```python
from build123d import *

# Parameters (mm, degrees)
BOSS_EXTRUDE1_DEPTH = 15
SKETCH3_R           = 1.5
CUT_EXTRUDE1_DEPTH  = 15


with BuildPart() as part:
    # Sketch2 → Boss-Extrude1 (new body)
    with BuildSketch(Plane(origin=(0, 0, 0), x_dir=(0, 0, -1), z_dir=(1, 0, 0))):
        with BuildLine():
            Line((8, 11.4), (-7.814981045, 11.4))
            Line((-7.814981045, 11.4), (-11.814981045, 11.4))
            Line((-11.814981045, 11.4), (-11.814981045, 9.4))
            Line((-11.814981045, 9.4), (-8, 9.4))
            Line((-8, 9.4), (-8, 0))
            ThreePointArc((-8, 0), (0, -8), (8, 0))
            Line((8, 0), (8, 9.4))
            Line((8, 9.4), (12, 9.4))
            Line((12, 9.4), (12, 11.4))
            Line((12, 11.4), (8, 11.4))
        make_face()
        with BuildLine():
            ThreePointArc((4, 0), (0, -4), (-4, 0))
            ThreePointArc((-4, 0), (0, 4), (4, 0))
        make_face(mode=Mode.SUBTRACT)
    extrude(amount=BOSS_EXTRUDE1_DEPTH)

    # Sketch3 → Cut-Extrude1 (cut)
    with BuildSketch(Plane.XZ.offset(-9.4)):
        with Locations(Location((2.464362638, -10, 0), (0, 0, 270))):
            Circle(SKETCH3_R)
        with Locations(Location((12.134124748, -10, 0), (0, 0, 270))):
            Circle(SKETCH3_R)
    cut_extrude1 = extrude(amount=-CUT_EXTRUDE1_DEPTH, mode=Mode.SUBTRACT)

    # Mirror1: Cut-Extrude1 across plane
    add(cut_extrude1.mirror(Plane.XY), mode=Mode.SUBTRACT)


solid = part.part
```
Build history of the part. All positions in model axes, mm. A direction names the side the tool comes from. Round coordinates to 2 decimals unless told otherwise and drop trailing zeros. Write each loop counter-clockwise with the first axis right and the second up, starting at its lowest first coordinate (ties: lowest second). Pieces come first, ordered by that corner, then holes.
1) Band-saw the part on B-B, the plane z = 0. List the corners of the cut face in (x, y).
2) 3-axis set-ups, long thin cutter, end or side, ignore diameter. For faces 4 (the flat face through (7, 9.4, -10)), 5 (the cylindrical face through (11.22, 10.39, -8.81)), 6 (the flat face through (7, 9.4, 10)): which of +Z, -Z, +X, -X, +Y, -Y reach the whole face in a straight line?
3) Band-saw the part on C-C, the plane x = 9.75. List the corners of the cut face in (y, z).
4) Band-saw the part on A-A, the plane z = 10. List the corners of the cut face in (x, y).
5) Mould opens along X. For faces 1 (the flat face through (0, 4, -3)), 2 (the flat face through (7, 5, -8)), 3 (the cylindrical face through (11.22, 10.39, 8.81)) say: +X half, -X half, draft (parallel to the pull), parting line (faces both ways), or undercut.
6) Drill centre lines: probe 1 along X at (y, z) = (10.2, 10); probe 2 along Y at (x, z) = (6.5, 0); probe 3 along Z at (x, y) = (13.25, 7.5). Where is each one in solid material? Low to high.
7) Pin check, flat tips, straight feed: pin 1 (2 mm diameter, centred on x = 9, z = -11, fed in from -Y); pin 2 (7 mm diameter, centred on y = 0, z = 0, fed in from -X) (1 decimal); pin 3 (4 mm diameter, centred on x = 1.5, y = -2.5, fed in from +Z); pin 4 (5 mm diameter, centred on x = 9.5, y = 2, fed in from -Z). Stop position of each tip, or through.
8) Band-saw the part on D-D, the plane y = 2. List the corners of the cut face in (x, z), and give its area (3 significant figures).
Ans:
1. outline: (0, -8) - (15, -8) - (15, -4) - (0, -4) - close; (0, 4) - (15, 4) - (15, 11.4) - (0, 11.4) - close
2. face 4: -Z, +X, -X, -Y
2. face 5: +Y, -Y
2. face 6: +Z, +X, -X, -Y
3. outline: (0, -8) - (9.4, -8) - (9.4, -12) - (11.4, -12) - (11.4, 11.81) - (9.4, 11.81) - (9.4, 8) - (0, 8) arc R8 ccw to start; hole circle Ø8 at (0, 0)
4. outline: (0, 9.4) - (0.96, 9.4) - (0.96, 11.4) - (0, 11.4) - close; (3.96, 9.4) - (10.63, 9.4) - (10.63, 11.4) - (3.96, 11.4) - close; (13.63, 9.4) - (15, 9.4) - (15, 11.4) - (13.63, 11.4) - close
5. face 1: -X half
5. face 2: draft
5. face 3: undercut
6. probe 1: x = 0 to 0.96, 3.96 to 10.63, 13.63 to 15
6. probe 2: y = -8 to -4, 4 to 11.4
6. probe 3: z = -8 to 8
7. pin 1: stops at y = 9.4
7. pin 2: passes through
7. pin 3: stops at z = 7.98
7. pin 4: stops at z = -8
8. outline: (0, -8) - (15, -8) - (15, -3.46) - (0, -3.46) - close; (0, 3.46) - (15, 3.46) - (15, 8) - (0, 8) - close
8. area: 136 mm2
